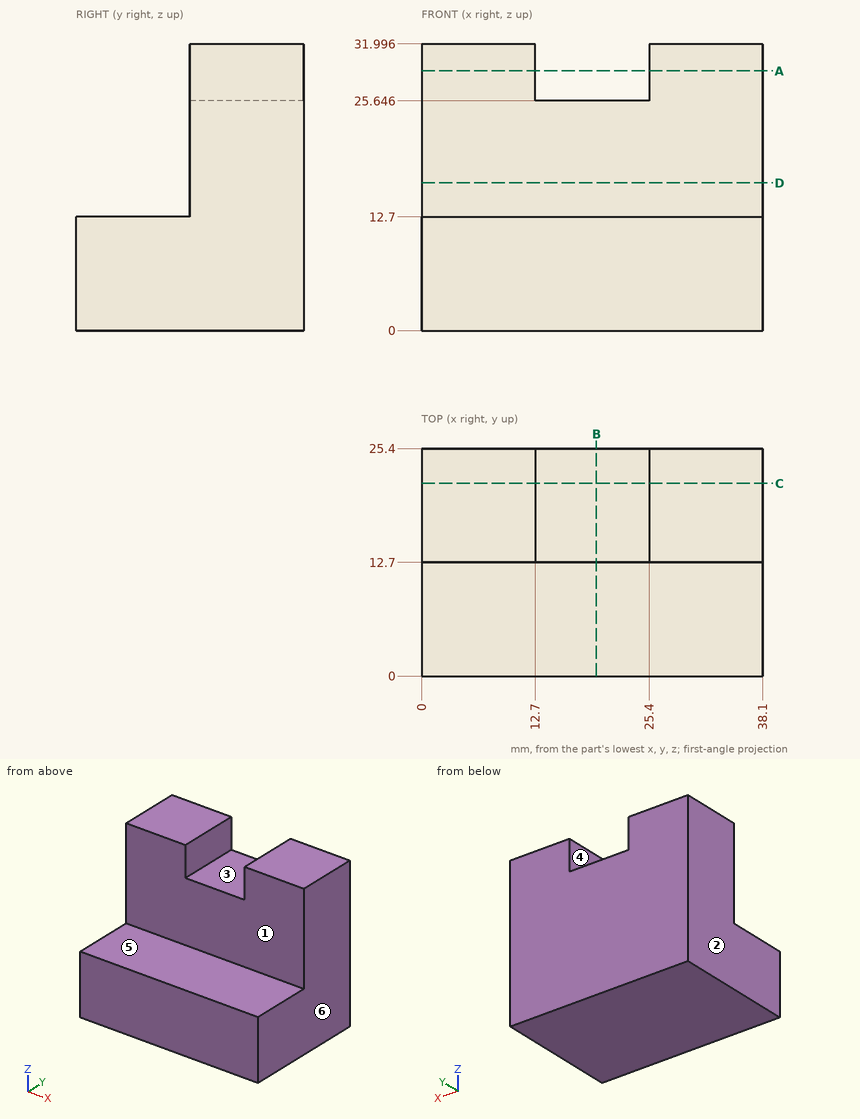
Geometry check sheet. Reference: drawing and pictorial views, mm from the part's lowest x, y, z. A direction names the side the tool comes from. Coordinates: 2 decimals unless noted, no trailing zeros. Write each loop counter-clockwise with the first axis right and the second up, starting at its lowest first coordinate (ties: lowest second). Pieces come first, ordered by that corner, then holes. Notation, with made-up numbers: (-36, -15.5) - (9, -15.5) arc R26 ccw to (9, 17.5) - close; hole circle Ø10 at (-12, 57). An arc over 180 degrees is marked (long way). One line per question, with ' | ' between items. Start each with the question number.
1. Section check A-A (z = 29). Enter the section's corners in (x, y), plus the area to 3 significant figures.
2. Section check D-D (z = 16.5). Enter the section's corners in (x, y), plus the area to 3 significant figures.
3. Section check C-C (y = 21.5). Enter the section's corners in (x, z) (1 decimal), plus the area to 3 significant figures.
4. Draft check along X on the marked faces 1, 2 and 3. Enter one of: released by +X, released by -X, zero draft, split by the parting line, or undercut.
5. Section check B-B (x = 19.5). Enter the section's corners in (y, z) (1 decimal).
6. Material ranges on line 1 along Y through (x, z) = (7.5, 26.5); line 2 along Z through (x, y) = (31.5, 8.75); line 3 along X through (y, z) = (19.25, 26), recorded low to high.
7. Access from +Z, -Z, +X, -X, +Y, -Y to the whole of each face (thin tool, end or side, straight path). Record for the marked faces 4, 5 and 6.
8. Gauge pin test, flat ends, axial feed: P1, Ø1.5, axis at x = 11.5, z = 17, coming from the -Y side; P2, Ø6.5, axis at x = 28, y = 8.5, coming from the +Z side; P3, Ø1, axis at x = 19.5, y = 18, coming from the +Z side. Record the tip position at first contact, or that the pin passes through.
Computed values:
1) outline: (0, 12.7) - (12.7, 12.7) - (12.7, 25.4) - (0, 25.4) - close; (25.4, 12.7) - (38.1, 12.7) - (38.1, 25.4) - (25.4, 25.4) - close | area: 323 mm²
2) outline: (0, 12.7) - (38.1, 12.7) - (38.1, 25.4) - (0, 25.4) - close | area: 484 mm²
3) outline: (0, 0) - (38.1, 0) - (38.1, 32) - (25.4, 32) - (25.4, 25.6) - (12.7, 25.6) - (12.7, 32) - (0, 32) - close | area: 1,140 mm²
4) face 1: zero draft | face 2: released by -X | face 3: undercut
5) outline: (0, 0) - (25.4, 0) - (25.4, 25.6) - (12.7, 25.6) - (12.7, 12.7) - (0, 12.7) - close
6) line 1: 12.7 to 25.4 | line 2: 0 to 12.7 | line 3: 0 to 12.7, 25.4 to 38.1
7) face 4: +Z, +Y, -Y | face 5: +Z, +X, -X, -Y | face 6: +Z, -Z, +X, +Y, -Y
8) P1: y = 12.7 | P2: z = 12.7 | P3: z = 25.65
